```python
from build123d import *

# Parameters (mm, degrees)
SKETCH1_W      = 10
SKETCH1_H      = 10
HEAD_DEPTH     = 3
SKETCH2_R      = 2
SHAFT_DEPTH    = 20.5
HEAD_FILLET_R  = 0.75
FILLET1_R      = 0.5
CHAMFER1_SIZE  = 0.5
CHAMFER1_SIZE2 = 0.288675135


with BuildPart() as part:
    # Sketch1 → head (new body)
    with BuildSketch(Plane(origin=(0, 0, 0), x_dir=(0, 0, -1), z_dir=(1, 0, 0))):
        Rectangle(SKETCH1_W, SKETCH1_H)
    extrude(amount=HEAD_DEPTH)

    # Sketch2 → shaft (add)
    with BuildSketch(Plane.ZY):
        with Locations(Location((0, 0, 0), (0, 0, 180))):  # turned: the seam where the file's is
            Circle(SKETCH2_R)
    extrude(amount=SHAFT_DEPTH)

    # head fillet
    head_fillet_edges = [part.edges().sort_by_distance(p)[0] for p in [
        (1.5, 5, 5),
        (1.5, 5, -5),
        (1.5, -5, -5),
        (1.5, -5, 5),
    ]]
    fillet(head_fillet_edges, radius=HEAD_FILLET_R)

    # Fillet1
    fillet1_edges = [part.edges().sort_by_distance(p)[0] for p in [
        (0, 0, 2),
    ]]
    fillet(fillet1_edges, radius=FILLET1_R)

    # Chamfer1
    chamfer1_edges = [part.edges().sort_by_distance(p)[0] for p in [
        (-20.5, 0, 2),
    ]]
    chamfer1_side = [part.faces().sort_by_distance(p)[0] for p in [
        (-20.5, 0, 0),
    ]]
    chamfer(chamfer1_edges, length=CHAMFER1_SIZE, length2=CHAMFER1_SIZE2, reference=chamfer1_side[0])


solid = part.part
```
Geometry: final body of the model. Coordinates: model frame, mm. A direction names the side the tool comes from. Coordinates: 2 decimals unless noted, no trailing zeros. Loops run counter-clockwise (first coordinate to the right, second up) from the corner with the lowest first, then second, coordinate; pieces in that order, holes last. Notation, with made-up numbers: (43, 3) -> (50, 3) arc R26 cw to (50, 19) -> close; hole circle Ø6 at (45.25, 26.25). An arc over 180 degrees is marked (long way). Use a Markdown table: item, result. Add a question column.
(1) Pin query (flat end, axial travel): pin 1 Ø2 at (y, z) = (3.5, -1.5) entering from -X; pin 2 Ø5 at (y, z) = (-1.5, 0.5) entering from -X. Return the tip coordinate at first contact, or that it passes through.
(2) Section query A-A, the plane z = 0. Return loops of the section in (x, y).
(3) Section query D-D, the plane y = -3. Return loops of the section in (x, z).
(4) Access query for faces 1 (the flat face through (-20.5, 0, 0)), 2 (the cylindrical face through (-10, 2, 0)). Directions: +Z, -Z, +X, -X, +Y, -Y. A direction counts if a zero-diameter tool reaches every point of the face in a straight line with its end or side. Return the directions, or none.
(5) Line query: line 1 along X through (y, z) = (0.5, 3.5); line 2 along Y through (x, z) = (-1.5, 0); line 3 along Z through (x, y) = (-8.75, 1.75). Output: solid intervals per line, ascending.
(6) Section query C-C, the plane x = -11.25. Return loops of the section in (y, z), plus the area to 3 significant figures.
Answer:
| question | item | result |
|---|---|---|
| 1 | pin 1 | stops at x = 0 |
| 1 | pin 2 | stops at x = -20.5 |
| 2 | outline | (-20.5, -1.5) -> (-20.21, -2) -> (-0.5, -2) arc R0.5 cw to (0, -2.5) -> (0, -5) -> (3, -5) -> (3, 5) -> (0, 5) -> (0, 2.5) arc R0.5 cw to (-0.5, 2) -> (-20.21, 2) -> (-20.5, 1.5) -> close |
| 3 | outline | (0, -5) -> (3, -5) -> (3, 5) -> (0, 5) -> close |
| 4 | face 1 | +Z, -Z, -X, +Y, -Y |
| 4 | face 2 | -X |
| 5 | line 1 | x = 0 to 3 |
| 5 | line 2 | y = -2 to 2 |
| 5 | line 3 | z = -0.97 to 0.97 |
| 6 | outline | circle Ø4 at (0, 0) |
| 6 | area | 12.6 mm^2 |
